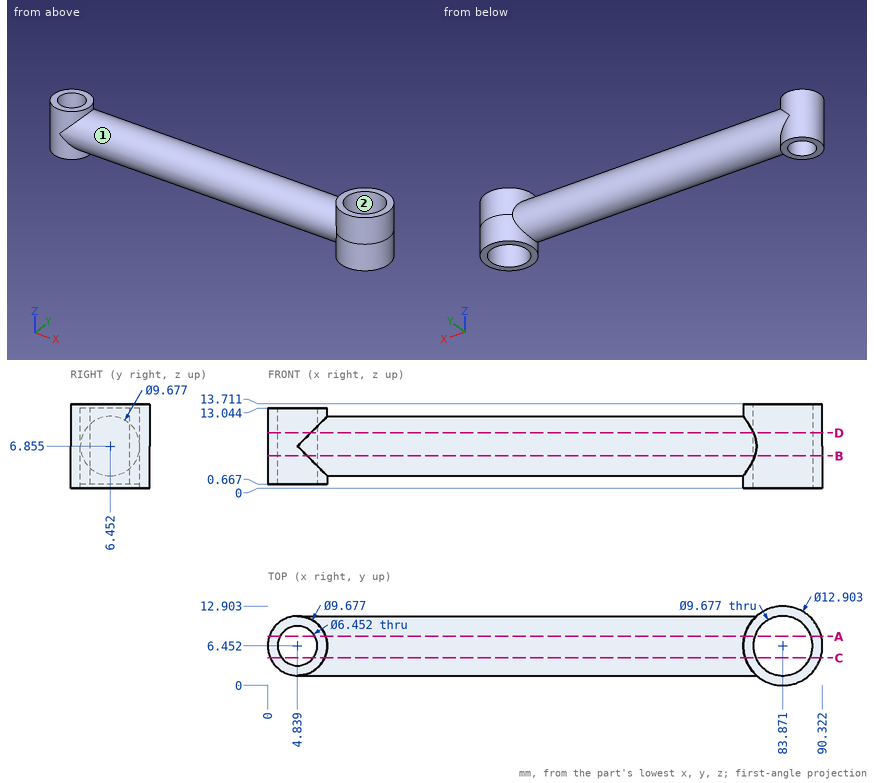
Design review of the part shown in the three views and the two pictorial views. Dimensions are in mm from the part's minimum x, y and z. Coordinates: 2 decimals unless noted, no trailing zeros. Loops run counter-clockwise (first coordinate to the right, second up) from the corner with the lowest first, then second, coordinate; pieces in that order, holes last. Notation, with made-up numbers: (-33, 89.5) - (18, 89.5) arc R33 ccw to (18, 121.5) - close; hole circle Ø6 at (42, -13.75). An arc over 180 degrees is marked (long way). Use a Markdown table: item, result. Add a question column.
Item 1: We need section B-B (z = 5.25). Give the boundary of the cut face in (x, y) (1 decimal).
Item 2: For line 1 (X direction, y = 6.25, z = 5) (1 decimal); line 2 (X direction, y = 8.75, z = 10.5) (1 decimal); line 3 (X direction, y = 7.5, z = 1.25) (1 decimal), list the stretches that pass through material, from the lowest coordinate up.
Item 3: We need section D-D (z = 9). Give the boundary of the cut face in (x, y) (1 decimal).
Item 4: Insertion check: pin 1 Ø2 at (x, y) = (56.5, 6) entering from -Z; pin 2 Ø6 at (x, y) = (77, 9.5) entering from -Z; pin 3 Ø5 at (x, y) = (7, 8.5) entering from -Z; pin 4 Ø6 at (x, y) = (59, 11) entering from +Z. Each pin has a flat end and moves straight along its axis. Give the tip position at first contact, or say it passes through.
Item 5: We need section C-C (y = 4.5). Give the boundary of the cut face in (x, z) (1 decimal).
Item 6: We need section A-A (y = 8). Give the boundary of the cut face in (x, z) (1 decimal).
Item 7: Mouldability with a two-part tool opening along Y and no side actions: class the marked faces 1 and 2 as pulls with the +Y half, pulls with the -Y half, needs draft (parallel to the pull), parting line crosses it, or undercut.
Results list:
| question | item | result |
|---|---|---|
| 1 | outline | (6.4, 1.9) - (79.3, 1.9) arc R6.5 ccw (long way) to (79.3, 11) - (6.4, 11) arc R4.8 ccw (long way) to start; hole circle Ø6.5 at (4.8, 6.5); hole circle Ø9.7 at (83.9, 6.5) |
| 2 | line 1 | x = 0 to 1.6, 8.1 to 79, 88.7 to 90.3 |
| 2 | line 2 | x = 0.6 to 2.6, 7.1 to 79.6, 88.1 to 89.9 |
| 2 | line 3 | x = 0.1 to 1.8, 7.9 to 9.6, 77.5 to 79.1, 88.6 to 90.2 |
| 3 | outline | (7, 2.1) - (79.1, 2.1) arc R6.5 ccw (long way) to (79.1, 10.8) - (7, 10.8) arc R4.8 ccw (long way) to start; hole circle Ø6.5 at (4.8, 6.5); hole circle Ø9.7 at (83.9, 6.5) |
| 4 | pin 1 | stops at z = 2.02 |
| 4 | pin 2 | stops at z = 0 |
| 4 | pin 3 | stops at z = 0.67 |
| 4 | pin 4 | stops at z = 11.44 |
| 5 | outline | (0.4, 0.7) - (2.3, 0.7) - (2.3, 13) - (0.4, 13) - close; (7.4, 0.7) - (9.3, 0.7) - (9.3, 2.4) - (77.7, 2.4) - (77.7, 0) - (79.4, 0) - (79.4, 13.7) - (77.7, 13.7) - (77.7, 11.3) - (9.3, 11.3) - (9.3, 13) - (7.4, 13) - close; (88.3, 0) - (90, 0) - (90, 13.7) - (88.3, 13.7) - close |
| 6 | outline | (0.3, 0.7) - (2, 0.7) - (2, 13) - (0.3, 13) - close; (7.7, 0.7) - (9.4, 0.7) - (9.4, 2.3) - (77.6, 2.3) - (77.6, 0) - (79.3, 0) - (79.3, 13.7) - (77.6, 13.7) - (77.6, 11.4) - (9.4, 11.4) - (9.4, 13) - (7.7, 13) - close; (88.5, 0) - (90.1, 0) - (90.1, 13.7) - (88.5, 13.7) - close |
| 7 | face 1 | parting line crosses it |
| 7 | face 2 | undercut |
